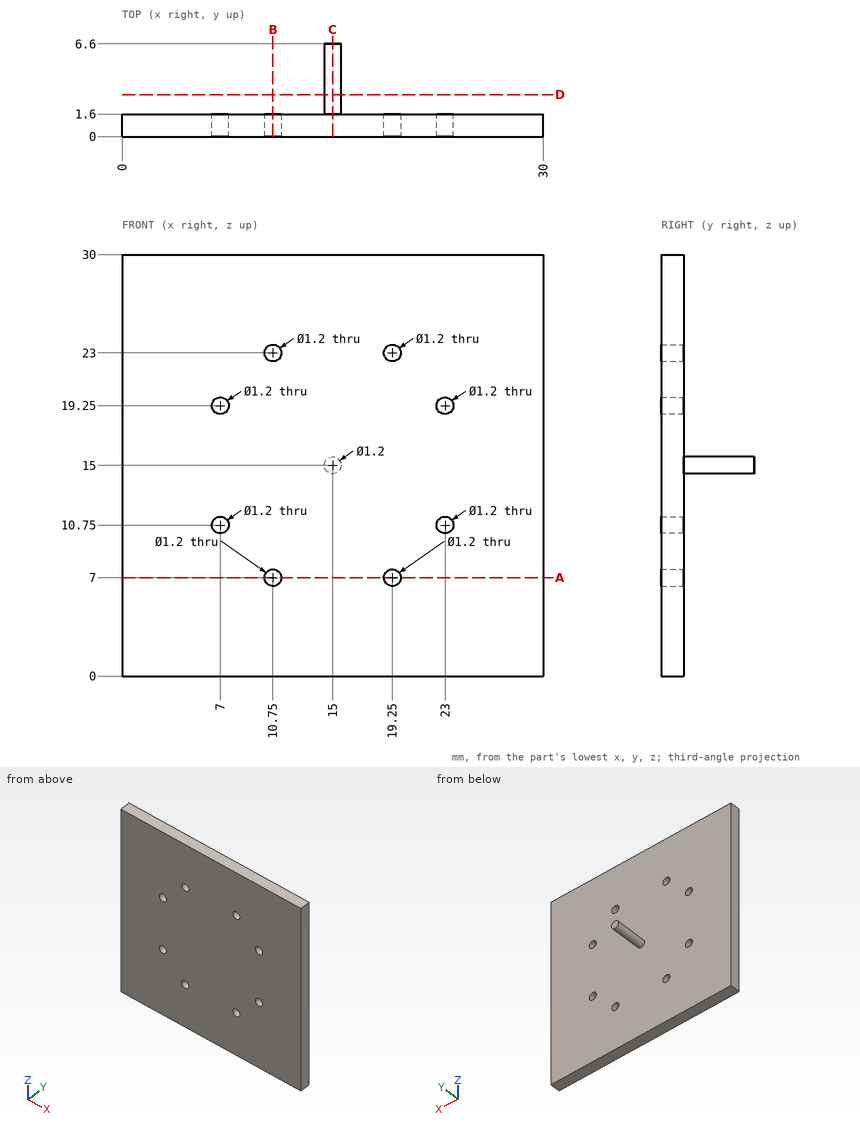
Answer from the drawing. Dimensions are ordinates in mm from the lowest x, y and z of the part. Round coordinates to 2 decimals unless told otherwise and drop trailing zeros. Order: outer loops, then holes, each group sorted by start corner. A loop starts at its lowest first (then second) coordinate and runs counter-clockwise, first axis right, second up. Notation, with made-up numbers: (-27, 4) - (14, 4) arc R24 cw to (14, 42) - close; hole circle Ø11 at (58, 38). An arc over 180 degrees is marked (long way). Put each result on its own line as item: value. Start each with the question number.
(1) Straight lines are drawn through the part: probe 1 along X at (y, z) = (0.8, 10.75); probe 2 along Z at (x, y) = (23, 1.1). For each, find the intervals that lie inside material, in ascending order. Write a range as from..to.
(2) Find section B-B (x = 10.75). Give the vertices of the cut face in (y, z).
(3) Given P1, Ø0.7, axis at x = 23, z = 19.25, coming from the -Y side; P2, Ø1.9, axis at x = 19.25, z = 23, coming from the +Y side, each flat-ended and moving along its own axis, determine where each tip first touches the part or whether it passes through.
(4) Find section C-C (x = 15). Give the vertices of the cut face in (y, z), plus the area to 3 significant figures.
(5) Find section D-D (y = 3). Give the vertices of the cut face in (x, z).
(6) Find section A-A (z = 7). Give the vertices of the cut face in (x, y).
Reply:
1. probe 1: 0..6.4, 7.6..22.4, 23.6..30
1. probe 2: 0..10.15, 11.35..18.65, 19.85..30
2. outline: (0, 0) - (1.6, 0) - (1.6, 6.4) - (0, 6.4) - close; (0, 7.6) - (1.6, 7.6) - (1.6, 22.4) - (0, 22.4) - close; (0, 23.6) - (1.6, 23.6) - (1.6, 30) - (0, 30) - close
3. P1: through
3. P2: y = 1.6
4. outline: (0, 0) - (1.6, 0) - (1.6, 14.4) - (6.6, 14.4) - (6.6, 15.6) - (1.6, 15.6) - (1.6, 30) - (0, 30) - close
4. area: 54.0 mm^2
5. outline: circle Ø1.2 at (15, 15)
6. outline: (0, 0) - (10.15, 0) - (10.15, 1.6) - (0, 1.6) - close; (11.35, 0) - (18.65, 0) - (18.65, 1.6) - (11.35, 1.6) - close; (19.85, 0) - (30, 0) - (30, 1.6) - (19.85, 1.6) - close
